Can you work these out from the model? Positions are in its coordinate system, mm. A direction names the side the tool comes from. Coordinates: 2 decimals unless noted, no trailing zeros. Loops run counter-clockwise (first coordinate to the right, second up) from the corner with the lowest first, then second, coordinate; pieces in that order, holes last.
```python
from build123d import *

# Parameters (mm, degrees)
BOSS_EXTRUDE1_DEPTH = 28
BOSS_EXTRUDE2_DEPTH = 2.5
BOSS_EXTRUDE3_START = -25.5
BOSS_EXTRUDE3_DEPTH = 2.5
CUT_EXTRUDE1_DEPTH  = 2.5
CUT_EXTRUDE2_DEPTH  = 2.5
BOSS_EXTRUDE4_DEPTH = 1
BOSS_EXTRUDE5_DEPTH = 1


with BuildPart() as part:
    # Sketch1 → Boss-Extrude1 (new body)
    with BuildSketch(Plane(origin=(0, 0, 0), x_dir=(1, 0, 0), z_dir=(0, 1, 0))):
        Polygon((0, 0), (0, 35), (2.5, 35), (2.5, 2.5), (35, 2.5), (35, 0), align=None)
    extrude(amount=BOSS_EXTRUDE1_DEPTH)

    # Sketch2 → Boss-Extrude2 (add)
    with BuildSketch(Plane(origin=(0, 28, 0), x_dir=(1, 0, 0), z_dir=(0, 1, 0))):
        with BuildLine():
            Line((2.5, 35), (4.25, 35))
            ThreePointArc((4.25, 35), (4.780330086, 34.780330086), (5, 34.25))
            Line((5, 34.25), (5, 32.5))
            Line((5, 32.5), (32.5, 5))
            Line((32.5, 5), (34.25, 5))
            ThreePointArc((34.25, 5), (34.780330086, 4.780330086), (35, 4.25))
            Line((35, 4.25), (35, 2.5))
            Line((35, 2.5), (2.5, 2.5))
            Line((2.5, 2.5), (2.5, 35))
        make_face()
    extrude(amount=-BOSS_EXTRUDE2_DEPTH)

    # Sketch2<2> → Boss-Extrude3 (add)
    with BuildSketch(Plane(origin=(0, 28, 0), x_dir=(1, 0, 0), z_dir=(0, 1, 0)).offset(BOSS_EXTRUDE3_START)):
        with BuildLine():
            Line((2.5, 35), (4.25, 35))
            ThreePointArc((4.25, 35), (4.780330086, 34.780330086), (5, 34.25))
            Line((5, 34.25), (5, 32.5))
            Line((5, 32.5), (32.5, 5))
            Line((32.5, 5), (34.25, 5))
            ThreePointArc((34.25, 5), (34.780330086, 4.780330086), (35, 4.25))
            Line((35, 4.25), (35, 2.5))
            Line((35, 2.5), (2.5, 2.5))
            Line((2.5, 2.5), (2.5, 35))
        make_face()
    extrude(amount=-BOSS_EXTRUDE3_DEPTH)

    # Sketch3 → Cut-Extrude1 (cut)
    with BuildSketch(Plane(origin=(0, 0, -2.5), x_dir=(-1, 0, 0), z_dir=(0, 0, -1))):
        with BuildLine():
            Line((-23.75, 17.5), (-13.75, 17.5))
            ThreePointArc((-13.75, 17.5), (-10.25, 14), (-13.75, 10.5))
            Line((-13.75, 10.5), (-23.75, 10.5))
            ThreePointArc((-23.75, 10.5), (-27.25, 14), (-23.75, 17.5))
        make_face()
    extrude(amount=-CUT_EXTRUDE1_DEPTH, mode=Mode.SUBTRACT)

    # Sketch4 → Cut-Extrude2 (cut)
    with BuildSketch(Plane(origin=(2.5, 0, 0), x_dir=(0, 0, -1), z_dir=(1, 0, 0))):
        with BuildLine():
            Line((13.75, 17.5), (23.75, 17.5))
            ThreePointArc((23.75, 17.5), (27.25, 14), (23.75, 10.5))
            Line((23.75, 10.5), (13.75, 10.5))
            ThreePointArc((13.75, 10.5), (10.25, 14), (13.75, 17.5))
        make_face()
    extrude(amount=-CUT_EXTRUDE2_DEPTH, mode=Mode.SUBTRACT)

    # Sketch5 → Boss-Extrude4 (add)
    with BuildSketch(Plane.XY):
        with BuildLine():
            Line((13.75, 18.5), (23.75, 18.5))
            ThreePointArc((23.75, 18.5), (28.25, 14), (23.75, 9.5))
            Line((23.75, 9.5), (13.75, 9.5))
            ThreePointArc((13.75, 9.5), (9.25, 14), (13.75, 18.5))
        make_face()
        with BuildLine():
            Line((13.75, 17.5), (23.75, 17.5))
            ThreePointArc((23.75, 17.5), (27.25, 14), (23.75, 10.5))
            Line((23.75, 10.5), (13.75, 10.5))
            ThreePointArc((13.75, 10.5), (10.25, 14), (13.75, 17.5))
        make_face(mode=Mode.SUBTRACT)
    extrude(amount=BOSS_EXTRUDE4_DEPTH)

    # Sketch6 → Boss-Extrude5 (add)
    with BuildSketch(Plane.ZY):
        with BuildLine():
            Line((-23.75, 18.5), (-13.75, 18.5))
            ThreePointArc((-13.75, 18.5), (-9.25, 14), (-13.75, 9.5))
            Line((-13.75, 9.5), (-23.75, 9.5))
            ThreePointArc((-23.75, 9.5), (-28.25, 14), (-23.75, 18.5))
        make_face()
        with BuildLine():
            Line((-13.75, 10.5), (-23.75, 10.5))
            ThreePointArc((-23.75, 10.5), (-27.25, 14), (-23.75, 17.5))
            Line((-23.75, 17.5), (-13.75, 17.5))
            ThreePointArc((-13.75, 17.5), (-10.25, 14), (-13.75, 10.5))
        make_face(mode=Mode.SUBTRACT)
    extrude(amount=BOSS_EXTRUDE5_DEPTH)


solid = part.part
```
Item 1: Suppose I cut it at B-B, the plane y = 14. Please give me the cut outline in (x, z).
Results are:
outline: (-1, -28.25) - (0, -28.25) - (0, -35) - (2.5, -35) - (2.5, -27.25) - (-1, -27.25) - close; (-1, -10.25) - (2.5, -10.25) - (2.5, -2.5) - (10.25, -2.5) - (10.25, 1) - (9.25, 1) - (9.25, 0) - (0, 0) - (0, -9.25) - (-1, -9.25) - close; (27.25, -2.5) - (35, -2.5) - (35, 0) - (28.25, 0) - (28.25, 1) - (27.25, 1) - close
Item 2: Suppose I cut it at A-A, the plane x = 22. Please give me the cut outline in (y, z).
Results are:
outline: (0, -15.5) - (2.5, -15.5) - (2.5, -2.5) - (10.5, -2.5) - (10.5, 1) - (9.5, 1) - (9.5, 0) - (0, 0) - close; (17.5, -2.5) - (25.5, -2.5) - (25.5, -15.5) - (28, -15.5) - (28, 0) - (18.5, 0) - (18.5, 1) - (17.5, 1) - close
Item 3: On a 3-axis mill with a long thin cutter (end or side, diameter ignored), from which of +Z, -Z, +X, -X, +Y, -Y can I reach the whole of each face in a straight line? I mean faces 5 (the face through (18.8, 9.5, 0.5)), 6 (the face through (10.25, 13.92, -0.77)), 7 (the face through (12, 2.5, -12)), 8 (the face through (1, 10.5, -19)), 9 (the face through (5, 1, -33)). Say none if no direction works.
Results are:
face 5: +Z, +X, -X, -Y
face 6: +Z, -Z
face 7: -Z, +X
face 8: +X, -X
face 9: -Z, +X, +Y, -Y
Item 4: We'd pull the mould along Z, two halves only. Please class faces 1 (the face through (0.77, 14.08, -10.25)), 2 (the face through (-0.49, 14.1, -9.25)), 3 (the face through (0.77, 13.92, -27.25)), 4 (the face through (9.25, 13.9, 0.49)): +Z half, -Z half, draft (parallel to the pull), parting line (faces both ways), or undercut.
Results are:
face 1: undercut
face 2: +Z half
face 3: undercut
face 4: draft
Item 5: I need wall thicknesses on line 1 along Y through (x, z) = (6.5, -3); line 2 along Z through (x, y) = (31, 3.25); line 3 along X through (y, z) = (6.25, -32.5). Which ranges of each line are inside material? Lowest first, please.
Results are:
line 1: y = 0 to 2.5, 25.5 to 28
line 2: z = -2.5 to 0
line 3: x = 0 to 2.5
Item 6: Suppose I cut it at D-D, the plane x = 8. Please give me the cut outline in (y, z).
Results are:
outline: (0, -29.5) - (2.5, -29.5) - (2.5, -2.5) - (25.5, -2.5) - (25.5, -29.5) - (28, -29.5) - (28, 0) - (0, 0) - close
Item 7: I'm going to push flat-ended pins straight in: P1, Ø1, axis at x = 14, y = 11.5, coming from the +Z side; P2, Ø1.4, axis at y = 27.5, z = -33, coming from the +X side; P3, Ø1.9, axis at x = 33, y = 1.5, coming from the -Z side; P4, Ø11.5, axis at x = 15, y = 16.5, coming from the -Z side. Where does each tip first touch, or does it pass through?
Results are:
P1: passes through
P2: stops at x = 5.2
P3: stops at z = -5.45
P4: stops at z = -2.5
Item 8: Suppose I cut it at C-C, the plane z = -25.5. Please give me the cut outline in (x, y), plus the area to 3 significant figures.
Results are:
outline: (-1, 9.85) - (0, 9.85) - (0, 0) - (12, 0) - (12, 2.5) - (2.5, 2.5) - (2.5, 10.97) - (-1, 10.97) - close; (-1, 17.03) - (2.5, 17.03) - (2.5, 25.5) - (12, 25.5) - (12, 28) - (0, 28) - (0, 18.15) - (-1, 18.15) - close
area: 105 mm2
